from build123d import *

# Parameters (mm, degrees)
EXTRUDE_1_DEPTH = 470


with BuildPart() as part:
    # 草图1 → 凸台-拉伸1 (new, symmetric)
    with BuildSketch(Plane.XY):
        Polygon((10.198060517, 15.211712223), (7.598340067, 18.189433578), (0, 18.189433578), (-7.598466158, 18.189433578), (-10.198186608, 15.211712223), (-10.198186608, 13.058876879), (-7.692519459, 10.438572741), (-7.692519459, 7.789953693), (-10, 5.165156487), (-10, 5.000194017), (-10, 0.355272087), (-9.644727913, 0), (-2.000943933, 0), (-1.650125997, 0.439438875), (1.650125997, 0.439438875), (2.000943933, 0), (9.644727913, 0), (10, 0.355272087), (10, 5.00019402), (10, 5.165156487), (7.692519459, 7.789953693), (7.692519459, 10.438572741), (10.198186608, 13.058876879), align=None)
    extrude(amount=EXTRUDE_1_DEPTH, both=True)


solid = part.part
For this review, take the finished solid that the model builds, in its own axes (mm). Round coordinates to 2 decimals unless told otherwise and drop trailing zeros. Order: outer loops, then holes, each group sorted by start corner. A loop starts at its lowest first (then second) coordinate and runs counter-clockwise, first axis right, second up. Notation, with made-up numbers: M 52.25,85.25 L 101.25,85.25 A16 ccw 101.25,98.25 Z; hole C 57,-32.5 d4. An arc over 180 degrees is marked long. Use a Markdown table: item, result. Add a question column.
Item 1: To check wall thickness, follow line 1 along X through (y, z) = (2.75, -148.5); line 2 along X through (y, z) = (15.5, -248.5); line 3 along Y through (x, z) = (1.5, 85.5). State the ranges of each line that lie inside material, in increasing order.
Item 2: Add section A-A, the plane z = -266. Give the boundary of the cut face in (x, y), then the cut area to 3 significant figures.
Item 3: Insertion check: pin 1 (2.5 mm diameter, centred on x = 0, z = 188, fed in from -Y); pin 2 (0.8 mm diameter, centred on y = 9, z = -119.5, fed in from +X); pin 3 (4 mm diameter, centred on y = 9, z = -61, fed in from -X). Each pin has a flat end and moves straight along its axis. Give the tip position at first contact, or say it passes through.
Geometry results:
| question | item | result |
|---|---|---|
| 1 | line 1 | x = -10 to 10 |
| 1 | line 2 | x = -9.95 to 9.95 |
| 1 | line 3 | y = 0.44 to 18.19 |
| 2 | outline | M -10.2,13.06 L -7.69,10.44 L -7.69,7.79 L -10,5.17 L -10,0.36 L -9.64,0 L -2,0 L -1.65,0.44 L 1.65,0.44 L 2,0 L 9.64,0 L 10,0.36 L 10,5.17 L 7.69,7.79 L 7.69,10.44 L 10.2,13.06 L 10.2,15.21 L 7.6,18.19 L -7.6,18.19 L -10.2,15.21 Z |
| 2 | area | 333 mm² |
| 3 | pin 1 | stops at y = 0.44 |
| 3 | pin 2 | stops at x = 7.69 |
| 3 | pin 3 | stops at x = -8.39 |
